from build123d import *

# Parameters (mm, degrees)
BODY_R          = 1.5
MAIN_BODY_DEPTH = 3
FIT_DEPTH       = 2


with BuildPart() as part:
    # body → main-body (new body)
    with BuildSketch(Plane.XY):
        with BuildLine():
            Line((-13.783032013, 30.826495293), (1.516967987, 30.826495293))
            ThreePointArc((1.516967987, 30.826495293), (8.981069602, 32.826495293), (3.516967987, 27.362393677))
            Line((3.516967987, 27.362393677), (-4.133032013, 14.112205))
            ThreePointArc((-4.133032013, 14.112205), (-6.133032013, 6.648103384), (-8.133032013, 14.112205))
            Line((-8.133032013, 14.112205), (-15.783032013, 27.362393677))
            ThreePointArc((-15.783032013, 27.362393677), (-21.247133628, 32.826495293), (-13.783032013, 30.826495293))
        make_face()
        with Locations((-17.783032013, 30.826495293)):
            Circle(BODY_R, mode=Mode.SUBTRACT)
        with Locations((5.516967987, 30.826495293)):
            Circle(BODY_R, mode=Mode.SUBTRACT)
        with Locations((-6.133032013, 10.648103384)):
            Circle(BODY_R, mode=Mode.SUBTRACT)
    extrude(amount=MAIN_BODY_DEPTH)

    # Skizze3 → fit (add)
    with BuildSketch(Plane.XY.offset(3)):
        Polygon((-11.958032013, 20.737299339), (-12.958032013, 22.469350146), (0.760919419, 30.389990449), (1.760919419, 28.657939641), align=None)
    extrude(amount=FIT_DEPTH)


solid = part.part
CAD build for the part. Positions are in the model's coordinates, mm. A direction names the side the tool comes from. Round coordinates to 2 decimals unless told otherwise and drop trailing zeros. Write each loop counter-clockwise with the first axis right and the second up, starting at its lowest first coordinate (ties: lowest second). Pieces come first, ordered by that corner, then holes. Notation, with made-up numbers: M 59,-37.75 L 97,-37.75 A28 ccw 97,-2.75 Z; hole C -20.5,1.5 d9. An arc over 180 degrees is marked long. Use a Markdown table: item, result. Add a question column.
1. 3-axis set-ups, long thin cutter, end or side, ignore diameter. For faces 1 (the face through (1.25, 29.54, 3.99)), 2 (the face through (-5.003, 24.753, 3.986)), 3 (the face through (-6, 24, 0)): which of +Z, -Z, +X, -X, +Y, -Y reach the whole face in a straight line?
2. Slice it at A-A on x = -8.5. Give the cut face in (y, z), then the cut area to 3 significant figures.
3. Slice it at D-D on x = -3.5. Give the cut face in (y, z), then the cut area to 3 significant figures.
4. Drill centre lines: probe 1 along X at (y, z) = (27.25, 2.3); probe 2 along X at (y, z) = (29.75, 1.95); probe 3 along X at (y, z) = (10.5, 2.8). Where is each one in solid material? Low to high.
5. Slice it at B-B on z = 0.4. Give the cut face in (x, y), then the cut area to 3 significant figures.
6. Slice it at C-C on y = 11.25. Give the cut face in (x, z).
7. Flat gauge pins, fed straight in: P1, Ø1.5, axis at x = -16, y = 28.5, coming from the +Z side; P2, Ø2.5, axis at x = -6.5, z = 2, coming from the +Y side. Where does each tip first touch, or does it go through?
8. Pull direction X, two halves, no side cores. Call faces 4 (the face through (-6, 24, 3)), 5 (the face through (-6.195, 26.374, 3.986)), 6 (the face through (-6, 30.826, 1)): released by +X, released by -X, zero draft, split by the parting line, or undercut.
Reply:
| question | item | result |
|---|---|---|
| 1 | face 1 | +Z, +X, +Y |
| 1 | face 2 | +Z, +X, -Y |
| 1 | face 3 | -Z, +X, -X, +Y, -Y |
| 2 | outline | M 7.42,0 L 13.87,0 L 13.87,3 L 7.42,3 Z; M 14.75,0 L 30.83,0 L 30.83,3 L 25.04,3 L 25.04,5 L 22.73,5 L 22.73,3 L 14.75,3 Z |
| 2 | area | 72.2 mm^2 |
| 3 | outline | M 7.64,0 L 13.66,0 L 13.66,3 L 7.64,3 Z; M 15.21,0 L 30.83,0 L 30.83,3 L 27.93,3 L 27.93,5 L 25.62,5 L 25.62,3 L 15.21,3 Z |
| 3 | area | 69.5 mm^2 |
| 4 | probe 1 | x = -19.57 to -15.99, -15.72 to 3.45, 3.73 to 7.31 |
| 4 | probe 2 | x = -21.64 to -18.83, -16.74 to 4.47, 6.56 to 9.37 |
| 4 | probe 3 | x = -10.13 to -7.63, -4.64 to -2.14 |
| 5 | outline | M -15.78,27.36 L -8.13,14.11 A4 ccw long -4.13,14.11 L 3.52,27.36 A4 ccw long 1.52,30.83 L -13.78,30.83 A4 ccw long Z; hole C -17.78,30.83 d3; hole C -6.13,10.65 d3; hole C 5.52,30.83 d3 |
| 5 | area | 340 mm^2 |
| 6 | outline | M -10.09,0 L -7.51,0 L -7.51,3 L -10.09,3 Z; M -4.76,0 L -2.18,0 L -2.18,3 L -4.76,3 Z |
| 7 | P1 | stops at z = 3 |
| 7 | P2 | stops at y = 30.83 |
| 8 | face 4 | zero draft |
| 8 | face 5 | released by -X |
| 8 | face 6 | undercut |
